Here's the drawing with two shaded views (mm, measured from the low corner). I have some questions. Coordinates: 2 decimals unless noted, no trailing zeros. Write each loop counter-clockwise with the first axis right and the second up, starting at its lowest first coordinate (ties: lowest second). Pieces come first, ordered by that corner, then holes.
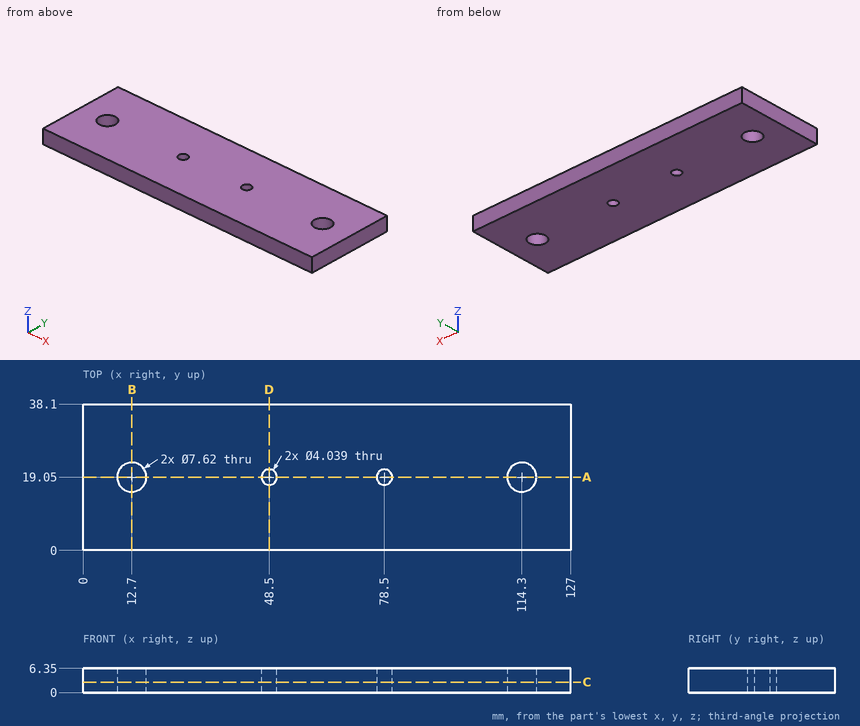
Item 1: I want a section at C-C, the plane z = 2.75. List the corners of the cut face in (x, y) for me.
Item 2: Will this pin go through, and if not, where does the flat tip stop? pin 1 Ø6 at (x, y) = (12.7, 19.05) entering from -Z.
Item 3: I want a section at B-B, the plane x = 12.7. List the corners of the cut face in (y, z) for me.
Item 4: I want a section at D-D, the plane x = 48.5. List the corners of the cut face in (y, z) for me, then the cut area to 3 significant figures.
Item 5: I want a section at A-A, the plane y = 19.05. List the corners of the cut face in (x, z) for me.
Item 6: If I drill on line 1 along Y through (x, z) = (114.3, 4.25); line 2 along Y through (x, z) = (114, 5), over which ranges is the centre line in solid material (lowest first)?
Taken from the geometry:
1. outline: (0, 0) - (127, 0) - (127, 38.1) - (0, 38.1) - close; hole circle Ø7.62 at (12.7, 19.05); hole circle Ø4.04 at (48.5, 19.05); hole circle Ø4.04 at (78.5, 19.05); hole circle Ø7.62 at (114.3, 19.05)
2. pin 1: passes through
3. outline: (0, 0) - (15.24, 0) - (15.24, 6.35) - (0, 6.35) - close; (22.86, 0) - (38.1, 0) - (38.1, 6.35) - (22.86, 6.35) - close
4. outline: (0, 0) - (17.03, 0) - (17.03, 6.35) - (0, 6.35) - close; (21.07, 0) - (38.1, 0) - (38.1, 6.35) - (21.07, 6.35) - close
4. area: 216 mm2
5. outline: (0, 0) - (8.89, 0) - (8.89, 6.35) - (0, 6.35) - close; (16.51, 0) - (46.48, 0) - (46.48, 6.35) - (16.51, 6.35) - close; (50.52, 0) - (76.48, 0) - (76.48, 6.35) - (50.52, 6.35) - close; (80.52, 0) - (110.49, 0) - (110.49, 6.35) - (80.52, 6.35) - close; (118.11, 0) - (127, 0) - (127, 6.35) - (118.11, 6.35) - close
6. line 1: y = 0 to 15.24, 22.86 to 38.1
6. line 2: y = 0 to 15.25, 22.85 to 38.1
